from build123d import *

# Parameters (mm, degrees)
SKETCH2_W                = 60
SKETCH2_H                = 120
BOSS_EXTRUDE1_DEPTH      = 60
SKETCH5_R                = 12.5
CUT_EXTRUDE2_DEPTH       = 48
BOSS_EXTRUDE3_DEPTH      = 20
BOSS_EXTRUDE3_DEPTH_BACK = 5
FILLET3_R                = 5
FILLET4_R                = 10
FILLET5_R                = 10
FILLET6_R                = 5
SKETCH7_R                = 12.5
BOSS_EXTRUDE4_DEPTH      = 50


with BuildPart() as part:
    # Sketch2 → Boss-Extrude1 (new body)
    with BuildSketch(Plane(origin=(0, 0, 0), x_dir=(0, 0, -1), z_dir=(1, 0, 0))):
        with Locations((0, 22.5)):
            Rectangle(SKETCH2_W, SKETCH2_H)
    extrude(amount=-BOSS_EXTRUDE1_DEPTH)

    # Sketch5 → Cut-Extrude2 (cut)
    with BuildSketch(Plane(origin=(0, 82.5, 0), x_dir=(1, 0, 0), z_dir=(0, 1, 0))):
        with Locations(Location((-30, 0, 0), (0, 0, 270))):
            Circle(SKETCH5_R)
    extrude(amount=-CUT_EXTRUDE2_DEPTH, mode=Mode.SUBTRACT)

    # Sketch6 → Boss-Extrude3 (add, two sides: drawn at the far end of the back side and taken through both)
    with BuildSketch(Plane.XY.offset(30).offset(-BOSS_EXTRUDE3_DEPTH_BACK)):
        with BuildLine():
            Line((0, 22.5), (0, -137.5))
            ThreePointArc((0, -137.5), (-30, -167.5), (-60, -137.5))
            Line((-60, -137.5), (-60, 22.5))
            ThreePointArc((-60, 22.5), (-30, 52.5), (0, 22.5))
        make_face()
    extrude(amount=BOSS_EXTRUDE3_DEPTH + BOSS_EXTRUDE3_DEPTH_BACK)

    # Fillet3
    fillet3_edges = [part.edges().sort_by_distance(p)[0] for p in [
        (-60, 52.5, 30),
        (-60, 22.5, -30),
        (0, 52.5, 30),
        (0, 82.5, 0),
        (0, 22.5, -30),
        (-60, 82.5, 0),
        (-30, 82.5, 30),
        (-30, 82.5, -30),
    ]]
    fillet(fillet3_edges, radius=FILLET3_R)


with BuildPart() as body_2:
    # Mirror2: mirrored copy
    add(part.part.mirror(Plane(origin=(0, 0, 0), x_dir=(1, 0, 0), z_dir=(0, 0, -1))))

    # Fillet5
    fillet5_edges = [body_2.edges().sort_by_distance(p)[0] for p in [
        (-30, 52.5, -50),
        (-60, -57.5, -50),
        (-30, -167.5, -50),
        (0, -57.5, -50),
    ]]
    fillet(fillet5_edges, radius=FILLET5_R)


with BuildPart() as part_1:
    add(part.part)

    # Fillet4
    fillet4_edges = [part_1.edges().sort_by_distance(p)[0] for p in [
        (-30, 52.5, 50),
        (-60, -57.5, 50),
        (-30, -167.5, 50),
        (0, -57.5, 50),
    ]]
    fillet(fillet4_edges, radius=FILLET4_R)

    # Fillet6
    fillet6_edges = [part_1.edges().sort_by_distance(p)[0] for p in [
        (0, -37.5, 0),
        (-60, -37.5, 0),
        (-30, -37.5, -30),
        (-58.535533906, -37.5, -28.535533906),
        (-1.464466094, -37.5, -28.535533906),
    ]]
    fillet(fillet6_edges, radius=FILLET6_R)

    add(body_2.part)  # Boss-Extrude4 merges body 2
    # Sketch7 → Boss-Extrude4 (add)
    with BuildSketch(Plane(origin=(0, 0, 25), x_dir=(-1, 0, 0), z_dir=(0, 0, -1))):
        with Locations(Location((30, -137.5, 0), (0, 0, 180))):
            Circle(SKETCH7_R)
    extrude(amount=BOSS_EXTRUDE4_DEPTH)


solid = part_1.part
Source: CAD feature listing. Evaluate the final solid. Frame: model axes, mm. A direction names the side the tool comes from. Give positions to 0.01 mm unless a question says otherwise; leave off trailing zeros. Order: outer loops, then holes, each group sorted by start corner. A loop starts at its lowest first (then second) coordinate and runs counter-clockwise, first axis right, second up. Notation, with made-up numbers: (32.25, -9.75) -> (48.25, -9.75) arc R4 ccw to (48.25, -4.75) -> close; hole circle Ø5 at (31.25, -9). An arc over 180 degrees is marked (long way). Use a Markdown table: item, result.
1) Reachability of faces 1 (the cylindrical face through (-1, 56, 28)), 2 (the cylindrical face through (-3.01, -58.62, -47.15)), 3 (the cylindrical face through (-1, 56, -28)) from +Z, -Z, +X, -X, +Y, -Y: full face, straight path, thin tool, end or side. Return the list, or none.
Answer list:
| item | result |
|---|---|
| face 1 | +Z, +X, +Y |
| face 2 | -Z, +X, +Y, -Y |
| face 3 | -Z, +X, +Y |
2) Ray query, line 1 along Z through (x, y) = (-30, 63.5); line 2 along X through (y, z) = (56, 0); line 3 along Z through (x, y) = (-34.5, -120.5). Return the intervals inside material, ascending. Write a range as [from, to].
Answer list:
| item | result |
|---|---|
| line 1 | [-30, -12.5], [12.5, 30] |
| line 2 | [-60, -42.5], [-17.5, 0] |
| line 3 | [-50, -25], [25, 50] |
3) Contact query for flat-ended pins moving along their axis: P1, Ø15, axis at x = -32, z = -5.5, coming from the -Y side; P2, Ø3, axis at x = -7, y = -142, coming from the +Z side; P3, Ø4, axis at x = -36.5, z = 1.5, coming from the -Y side; P4, Ø4, axis at x = -10.5, z = -27, coming from the +Y side. Output: stop coordinate, or through.
Answer list:
| item | result |
|---|---|
| P1 | y = -150 |
| P2 | z = 49.81 |
| P3 | y = -149.16 |
| P4 | y = 82.5 |
4) Section query D-D, the plane z = -32.5. Return the cut outline in (x, y), then the cut area to 3 significant figures.
Answer list:
| item | result |
|---|---|
| outline | (-60, -137.5) arc R30 ccw to (0, -137.5) -> (0, 22.5) arc R30 ccw to (-60, 22.5) -> close |
| area | 12,400 mm² |
5) Section query A-A, the plane y = -59. Return the cut outline in (x, z).
Answer list:
| item | result |
|---|---|
| outline | (-60, -40) arc R10 ccw to (-50, -50) -> (-10, -50) arc R10 ccw to (0, -40) -> (0, -25) -> (-60, -25) -> close; (-60, 25) -> (0, 25) -> (0, 40) arc R10 ccw to (-10, 50) -> (-50, 50) arc R10 ccw to (-60, 40) -> close |
6) Mould query, pull axis Y, two halves, no side actions, for faces 4 (the flat face through (0, -28, -1)), 5 (the cylindrical face through (-30.66, 52.493, 34.062)), 6 (the cylindrical face through (-29.34, -167.493, -32.395)), 7 (the flat face through (-30, -37.5, 0)). Classes: +Y half, -Y half, draft (parallel to the pull), parting line (faces both ways), or undercut.
Answer list:
| item | result |
|---|---|
| face 4 | draft |
| face 5 | +Y half |
| face 6 | -Y half |
| face 7 | undercut |
7) Section query B-B, the plane z = 0. Return the cut outline in (x, y).
Answer list:
| item | result |
|---|---|
| outline | (-60, -37.5) -> (0, -37.5) -> (0, 77.5) arc R5 ccw to (-5, 82.5) -> (-17.5, 82.5) -> (-17.5, 34.5) -> (-42.5, 34.5) -> (-42.5, 82.5) -> (-55, 82.5) arc R5 ccw to (-60, 77.5) -> close; circle Ø25 at (-30, -137.5) |
8) Section query C-C, the plane x = -30. Return the cut outline in (y, z).
Answer list:
| item | result |
|---|---|
| outline | (-167.5, -40) arc R10 ccw to (-157.5, -50) -> (42.5, -50) arc R10 ccw to (52.5, -40) -> (52.5, -30) -> (77.5, -30) arc R5 ccw to (82.5, -25) -> (82.5, -12.5) -> (34.5, -12.5) -> (34.5, 12.5) -> (82.5, 12.5) -> (82.5, 25) arc R5 ccw to (77.5, 30) -> (52.5, 30) -> (52.5, 40) arc R10 ccw to (42.5, 50) -> (-157.5, 50) arc R10 ccw to (-167.5, 40) -> (-167.5, 25) -> (-150, 25) -> (-150, -25) -> (-167.5, -25) -> close; hole (-125, -25) -> (-37.5, -25) -> (-37.5, 25) -> (-125, 25) -> close |
